Geometry: see drawing. Coordinates: mm, zero at the bounding-box minimum. A direction names the side the tool comes from. Coordinates: 2 decimals unless noted, no trailing zeros. Loops run counter-clockwise (first coordinate to the right, second up) from the corner with the lowest first, then second, coordinate; pieces in that order, holes last. Notation, with made-up numbers: (51, 53) - (74, 53) arc R7 ccw to (74, 62) - close; hole circle Ø8 at (-18.75, 28). An arc over 180 degrees is marked (long way). Use a Markdown table: item, result. Add a question column.
1. Section query C-C on z = 9.5. Return the cut outline in (x, y) (3 decimals), then the cut area to 3 significant figures.
2. Section query D-D on y = 13. Return the cut outline in (x, z) (3 decimals), then the cut area to 3 significant figures.
3. Contact query for flat-ended pins moving along their axis: P1, Ø8, axis at x = 15, y = 6.5, coming from the +Z side; P2, Ø5, axis at x = 21.5, z = 4.5, coming from the -Y side; P3, Ø5, axis at x = 3, z = 1.5, coming from the -Y side; P4, Ø5.5, axis at x = 8, y = 8, coming from the -Z side. Output: stop coordinate, or through.
4. Access query for the marked faces 1, 2 and 3. Directions: +Z, -Z, +X, -X, +Y, -Y. A direction counts if a zero-diameter tool reaches every point of the face in a straight line with its end or side. Return the directions, or none.
5. Ray query, L1, parallel to Y at x = 8, z = 0.85; L2, parallel to X at y = 8, z = 0.3; L3, parallel to Y at x = 8, z = 2.25. Return the intervals inside material, ascending. Write a range as [from, to].
6. Section query B-B on y = 6.75. Return the cut outline in (x, z), then the cut area to 3 significant figures.
7. Section query A-A on x = 25.2. Return the cut outline in (y, z) (3 decimals).
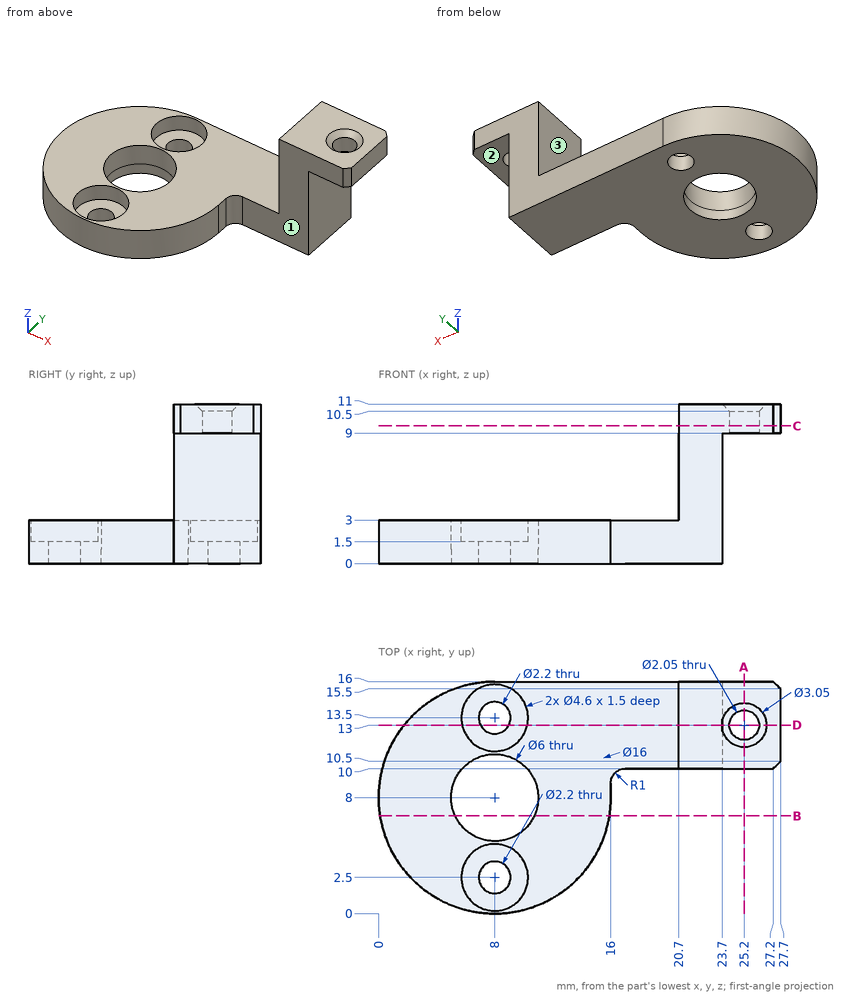
Resolved:
| question | item | result |
|---|---|---|
| 1 | outline | (20.7, 10) - (27.2, 10) - (27.7, 10.5) - (27.7, 15.5) - (27.2, 16) - (20.7, 16) - close; hole circle Ø2.05 at (25.2, 13) |
| 1 | area | 38.4 mm² |
| 2 | outline | (1.755, 0) - (7.02, 0) - (7.02, 1.5) - (5.755, 1.5) - (5.755, 3) - (1.755, 3) - close; (8.98, 0) - (23.7, 0) - (23.7, 9) - (24.175, 9) - (24.175, 10.5) - (23.675, 11) - (20.7, 11) - (20.7, 3) - (10.245, 3) - (10.245, 1.5) - (8.98, 1.5) - close; (26.225, 9) - (27.7, 9) - (27.7, 11) - (26.725, 11) - (26.225, 10.5) - close |
| 2 | area | 83.8 mm² |
| 3 | P1 | z = 3 |
| 3 | P2 | y = 10 |
| 3 | P3 | y = 0.4 |
| 3 | P4 | through |
| 4 | face 1 | +Z, -Z, +X, -Y |
| 4 | face 2 | -Z, +X, +Y, -Y |
| 4 | face 3 | +Z, -X, +Y, -Y |
| 5 | L1 | [0, 1.4], [3.6, 5], [11, 12.4], [14.6, 16] |
| 5 | L2 | [0, 5], [11, 16] |
| 5 | L3 | [0, 0.2], [4.8, 5], [11, 11.2], [15.8, 16] |
| 6 | outline | (0.1, 0) - (5.27, 0) - (5.27, 3) - (0.1, 3) - close; (10.73, 0) - (15.9, 0) - (15.9, 3) - (10.73, 3) - close |
| 6 | area | 31.0 mm² |
| 7 | outline | (10, 9) - (11.975, 9) - (11.975, 10.5) - (11.475, 11) - (10, 11) - close; (14.025, 9) - (16, 9) - (16, 11) - (14.525, 11) - (14.025, 10.5) - close |
